from build123d import *

# Parameters (mm, degrees)
SKETCH1_R           = 19.8
BOSS_EXTRUDE1_DEPTH = 2
SKETCH2_R           = 1.5
CUT_EXTRUDE1_DEPTH  = 5
SKETCH3_R           = 10
BOSS_EXTRUDE2_DEPTH = 100
SKETCH4_R           = 6
CUT_EXTRUDE3_DEPTH  = 200
SKETCH6_R           = 8
CUT_EXTRUDE4_DEPTH  = 10
SKETCH13_R          = 2
CUT_EXTRUDE7_DEPTH  = 20


with BuildPart() as part:
    # Sketch1 → Boss-Extrude1 (new body)
    with BuildSketch(Plane.XY):
        Circle(SKETCH1_R)
    extrude(amount=BOSS_EXTRUDE1_DEPTH)

    # Sketch2 → Cut-Extrude1 (cut)
    with BuildSketch(Plane.XY.offset(2)):
        with Locations((0, 15)):
            Circle(SKETCH2_R)
        with Locations((15, 0)):
            Circle(SKETCH2_R)
        with Locations((0, -15)):
            Circle(SKETCH2_R)
        with Locations((-15, 0)):
            Circle(SKETCH2_R)
    extrude(amount=-CUT_EXTRUDE1_DEPTH, mode=Mode.SUBTRACT)

    # Sketch3 → Boss-Extrude2 (add)
    with BuildSketch(Plane.XY.offset(2)):
        Circle(SKETCH3_R)
    extrude(amount=BOSS_EXTRUDE2_DEPTH)

    # Sketch4 → Cut-Extrude3 (cut)
    with BuildSketch(Plane.XY.offset(102)):
        Circle(SKETCH4_R)
    extrude(amount=-CUT_EXTRUDE3_DEPTH, mode=Mode.SUBTRACT)

    # Sketch6 → Cut-Extrude4 (cut)
    with BuildSketch(Plane.XY.offset(102)):
        Circle(SKETCH6_R)
    extrude(amount=-CUT_EXTRUDE4_DEPTH, mode=Mode.SUBTRACT)

    # Sketch13 → Cut-Extrude7 (cut)
    with BuildSketch(Plane(origin=(0, 10, 0), x_dir=(1, 0, 0), z_dir=(0, 1, 0))):
        with Locations(Location((0, -97, 0), (0, 0, 270))):
            Circle(SKETCH13_R)
    extrude(amount=-CUT_EXTRUDE7_DEPTH, mode=Mode.SUBTRACT)


solid = part.part
Geometry: final body of the model. Coordinates: model frame, mm. A direction names the side the tool comes from. Give positions to 0.01 mm unless a question says otherwise; leave off trailing zeros. Loops run counter-clockwise (first coordinate to the right, second up) from the corner with the lowest first, then second, coordinate; pieces in that order, holes last. Notation, with made-up numbers: M 77.5,83.25 L 104.5,83.25 A18 cw 104.5,100.25 Z; hole C -8,46 d3. An arc over 180 degrees is marked long. Put each result on its own line as item: value. Start each with the question number.
1) Contact query for flat-ended pins moving along their axis: pin 1 (5 mm diameter, centred on x = 0, z = 97, fed in from +Y); pin 2 (6 mm diameter, centred on x = -6, z = 27.5, fed in from +Y); pin 3 (12 mm diameter, centred on y = -15, z = 81, fed in from +X). Output: stop coordinate, or through.
2) Cut plane B-B (x = 0). Give the number of separate pieces and of enclosed holes in the cut face, then the cut area to 3 significant figures.
3) Ray query, line 1 along X through (y, z) = (8, 97); line 2 along Y through (x, z) = (0, 71); line 3 along Z through (x, y) = (2.5, -11.5). Return the intervals inside material, ascending.
4) Pull-direction query (X, two-part tool) for faces 1 (the cylindrical face through (1.352, 8.889, 95.526)), 2 (the cylindrical face through (18.9, 5.9, 1)), 3 (the flat face through (-5, -4, 0)); classes: pulls with the +X half, pulls with the -X half, needs draft (parallel to the pull), parting line crosses it, or undercut.
5) Access query for faces 4 (the cylindrical face through (-16.5, 0.07, 1.01)), 5 (the cylindrical face through (3.69, -7.1, 97.07)). Directions: +Z, -Z, +X, -X, +Y, -Y. A direction counts if a zero-diameter tool reaches every point of the face in a straight line with its end or side. Return the directions, or none.
6) Cut plane A-A (y = 0). Output: boundary loops of the cut face in (x, z), then the cut area to 3 significant figures.
7) Cut plane C-C (z = 97). Output: boundary loops of the cut face in (x, y).
8) Cut plane D-D (x = 14.5). Output: boundary loops of the cut face in (y, z).
Verdict:
1. pin 1: y = 10
1. pin 2: y = 9.54
1. pin 3: x = 4.36
2. separate pieces: 6
2. enclosed holes: 0
2. area: 787 mm2
3. line 1: -6 to -2, 2 to 6
3. line 2: -10 to -6, 6 to 10
3. line 3: 0 to 2
4. face 1: undercut
4. face 2: parting line crosses it
4. face 3: needs draft
5. face 4: +Z, -Z
5. face 5: +Z
6. outline: M -19.8,0 L -16.5,0 L -16.5,2 L -19.8,2 Z; M -13.5,0 L -6,0 L -6,92 L -8,92 L -8,102 L -10,102 L -10,2 L -13.5,2 Z; M 6,0 L 13.5,0 L 13.5,2 L 10,2 L 10,102 L 8,102 L 8,92 L 6,92 Z; M 16.5,0 L 19.8,0 L 19.8,2 L 16.5,2 Z
6. area: 803 mm2
7. outline: M -2,-9.8 L -2,-7.75 A8 cw -2,7.75 L -2,9.8 A10 ccw Z; M 2,-9.8 A10 ccw 2,9.8 L 2,7.75 A8 cw 2,-7.75 Z
8. outline: M -13.48,0 L -1.41,0 L -1.41,2 L -13.48,2 Z; M 1.41,0 L 13.48,0 L 13.48,2 L 1.41,2 Z
